Autodesk Inventor part; units mm, degrees
ref_plane "YZ Plane" through (0, 0, 0) normal (1, 0, 0) x (0, 1, 0)
ref_plane "XZ Plane" through (0, 0, 0) normal (0, 1, 0) x (-1, 0, 0)
ref_plane "XY Plane" through (0, 0, 0) normal (0, 0, 1) x (1, 0, 0)
sketch "Sketch1" plane through (0, 0, 0) normal (0, 1, 0) x (-1, 0, 0)
  line L0 (0, 0) -> (10, 0)
  line L1 (10, 0) -> (10, -165)
  line L2 (10, -165) -> (0, -165)
  line L3 (0, -165) -> (0, 0)
  dimension "d0" = 10
  dimension "d1" = 165
extrude "Extrusion1" add sketch "Sketch1" along normal blind 200
sketch "Sketch2" plane through (-10, 0, 0) normal (0, 0, 1) x (1, 0, 0)
  line L0 (2.5, 15) -> (7.5, 15)
  line L1 (7.5, 15) -> (7.5, 185)
  line L2 (7.5, 185) -> (2.5, 185)
  line L3 (2.5, 185) -> (2.5, 15)
  point P0 (10, 0)
  dimension "d4" = 5
  dimension "d5" = 170
extrude "Extrusion2" add sketch "Sketch2" along normal blind 25
sketch "Sketch3" plane through (0, 0, -165) normal (0, 0, -1) x (-1, 0, 0)
  line L0 (2.5, 15) -> (7.5, 15)
  line L1 (7.5, 15) -> (7.5, 185)
  line L2 (7.5, 185) -> (2.5, 185)
  line L3 (2.5, 185) -> (2.5, 15)
  point P0 (0, 0)
  dimension "d8" = 5
  dimension "d9" = 170
extrude "Extrusion3" cut sketch "Sketch3" against normal blind 25
sketch "Sketch4" plane through (-10, 0, -165) normal (-1, 0, 0) x (0, 0, 1)
  line L0 (0, 200) -> (165, 200) construction
  line L1 (82.5, 200) -> (82.5, 0) construction
  line L2 (0, 0) -> (165, 0) construction
  line L3 (107.5, 175) -> (132.5, 175)
  line L4 (132.5, 175) -> (132.5, 25)
  line L5 (132.5, 25) -> (107.5, 25)
  line L6 (107.5, 25) -> (107.5, 175)
  line L7 (57.5, 175) -> (32.5, 175)
  line L8 (32.5, 175) -> (32.5, 25)
  line L9 (32.5, 25) -> (57.5, 25)
  line L10 (57.5, 25) -> (57.5, 175)
  dimension "d12" = 25
  dimension "d13" = 150
  dimension "d14" = 25
  dimension "d15" = 150
extrude "Extrusion4" cut sketch "Sketch4" against normal blind 10
fillet "Fillet1" radius 12.5 8 edges at (-5, 175, -107.5) (-5, 175, -32.5) (-5, 175, -57.5) (-5, 175, -132.5) (-5, 25, -132.5) (-5, 25, -107.5) (-5, 25, -57.5) (-5, 25, -32.5)
properties part number "TSU_FM_Side_Wall"
Read the model definition and answer for the solid it produces. Units are mm, in the model's axes. A direction names the side the tool comes from. Round coordinates to 2 decimals unless told otherwise and drop trailing zeros. Write each loop counter-clockwise with the first axis right and the second up, starting at its lowest first coordinate (ties: lowest second). Pieces come first, ordered by that corner, then holes. Notation, with made-up numbers: (-25.75, -30.75) -> (-14.75, -30.75) arc R22 ccw to (-14.75, -0.75) -> close; hole circle Ø10 at (-7, 32). An arc over 180 degrees is marked (long way). Answer in a Markdown table with one row per item. Add a question column.
1) Which of the six approach directions +Z, -Z, +X, -X, +Y, -Y give full straight-line access (tool end or side, diameter ignored) to faces 1 (the face through (-5, 185, -153)), 2 (the face through (-2.5, 99, 12)), 3 (the face through (-5, 185, 12)), 4 (the face through (-5, 200, -81)), 5 (the face through (-5, 99, -107.5))?
2) Find section D-D, the plane y = 165. Determine the outline of the cut face in (x, z).
3) Determine the mould class of faces 6 (the face through (-8, 99, -165)), 7 (the face through (-4.93, 28.759, -111.064)), 8 (the face through (-2.5, 101, -153)) for opening direction Z: pulls with the +Z half, pulls with the -Z half, needs draft (parallel to the pull), parting line crosses it, or undercut.
4) Find section A-A, the plane y = 107. Determine the outline of the cut face in (x, z).
5) Given P1, Ø20, axis at y = 95, z = 12.5, coming from the +X side; P2, Ø3, axis at x = -5, y = 112, coming from the -Z side; P3, Ø4, axis at x = -6, z = 9, coming from the -Y side; P4, Ø4, axis at y = 35.5, z = -110.5, coming from the -X side, each flat-ended and moving along its own axis, determine where each tip first touches the part or whether it passes through.
6) Consider line 1 (Z direction, x = -1, y = 154); line 2 (Z direction, x = -3.5, y = 161); line 3 (X direction, y = 48.5, z = -154.5). Determine where each line is inside the solid, lowest interval first.
7) Find section B-B, the plane z = -52. Determine the outline of the cut face in (x, y), and give its area (3 significant figures).
8) Find section C-C, the plane x = -5. State how many separate pieces and enclosed holes the cut face has, and give its area (3 significant figures).
Findings below:
| question | item | result |
|---|---|---|
| 1 | face 1 | -Z |
| 1 | face 2 | +Z, +X, +Y, -Y |
| 1 | face 3 | +Z, +X, -X, +Y |
| 1 | face 4 | +Z, -Z, +X, -X, +Y |
| 1 | face 5 | +X, -X |
| 2 | outline | (-10, -165) -> (-7.5, -165) -> (-7.5, -140) -> (-2.5, -140) -> (-2.5, -165) -> (0, -165) -> (0, -132.25) -> (-10, -132.25) -> close; (-10, -107.75) -> (0, -107.75) -> (0, -57.25) -> (-10, -57.25) -> close; (-10, -32.75) -> (0, -32.75) -> (0, 0) -> (-2.5, 0) -> (-2.5, 25) -> (-7.5, 25) -> (-7.5, 0) -> (-10, 0) -> close |
| 3 | face 6 | pulls with the -Z half |
| 3 | face 7 | undercut |
| 3 | face 8 | needs draft |
| 4 | outline | (-10, -165) -> (-7.5, -165) -> (-7.5, -140) -> (-2.5, -140) -> (-2.5, -165) -> (0, -165) -> (0, -132.5) -> (-10, -132.5) -> close; (-10, -107.5) -> (0, -107.5) -> (0, -57.5) -> (-10, -57.5) -> close; (-10, -32.5) -> (0, -32.5) -> (0, 0) -> (-2.5, 0) -> (-2.5, 25) -> (-7.5, 25) -> (-7.5, 0) -> (-10, 0) -> close |
| 5 | P1 | x = -2.5 |
| 5 | P2 | z = -140 |
| 5 | P3 | y = 15 |
| 5 | P4 | through |
| 6 | line 1 | -165 to -132.5, -107.5 to -57.5, -32.5 to 0 |
| 6 | line 2 | -140 to -132.5, -107.5 to -57.5, -32.5 to 25 |
| 6 | line 3 | -10 to -7.5, -2.5 to 0 |
| 7 | outline | (-10, 0) -> (0, 0) -> (0, 27.14) -> (-10, 27.14) -> close; (-10, 172.86) -> (0, 172.86) -> (0, 200) -> (-10, 200) -> close |
| 7 | area | 543 mm² |
| 8 | separate pieces | 1 |
| 8 | enclosed holes | 2 |
| 8 | area | 25,800 mm² |
